from build123d import *

# Parameters (mm, degrees)
F0_W     = 50.8
F0_H     = 736.6
F1_DEPTH = 609.6
F2_W     = 685.8
F2_H     = 558.8
F3_DEPTH = 50.8
F4_W     = 25.4
F4_H     = 609.6
F5_DEPTH = 50.8


with BuildPart() as f1:
    # F0 (on Top) → F1 (new body)
    with BuildSketch(Plane.XY):
        with Locations((-589.687777, 189.852441)):
            Rectangle(F0_W, F0_H)
    extrude(amount=F1_DEPTH)

    # F2 (on face) → F3 (cut)
    with BuildSketch(Plane(origin=(-615.087777, 0, 0), x_dir=(0, -1, 0), z_dir=(-1, 0, 0))):
        with Locations((-189.852441, 304.8)):
            Rectangle(F2_W, F2_H)
    extrude(amount=-F3_DEPTH, mode=Mode.SUBTRACT)

    # F4 (on face) → F5 (cut)
    with BuildSketch(Plane(origin=(-615.087777, 0, 0), x_dir=(0, -1, 0), z_dir=(-1, 0, 0))):
        with Locations((165.747559, 304.8)):
            Rectangle(F4_W, F4_H)
    extrude(amount=-F5_DEPTH, mode=Mode.SUBTRACT)


solid = f1.part
Design review of the part built by this model. Coordinates are the model's own, in mm. A direction names the side the tool comes from. Round coordinates to 2 decimals unless told otherwise and drop trailing zeros. Order: outer loops, then holes, each group sorted by start corner. A loop starts at its lowest first (then second) coordinate and runs counter-clockwise, first axis right, second up.
1) Consider section A-A (y = 333). State the section outline as (x, z) points.
The answers:
outline: (-615.09, 0) - (-564.29, 0) - (-564.29, 25.4) - (-615.09, 25.4) - close; (-615.09, 584.2) - (-564.29, 584.2) - (-564.29, 609.6) - (-615.09, 609.6) - close
2) Consider section B-B (x = -574.5). State the section outline as (y, z) points.
The answers:
outline: (-153.05, 0) - (558.15, 0) - (558.15, 609.6) - (-153.05, 609.6) - (-153.05, 584.2) - (532.75, 584.2) - (532.75, 25.4) - (-153.05, 25.4) - close
3) Machinability: for faces 1 (the flat face through (-615.088, 543, 303)), 2 (the flat face through (-590, 532.752, 301)), which of the approach directions +Z, -Z, +X, -X, +Y, -Y give a long, thin tool a straight path to every point of the face, cutting with its end or side? Answer none if there is none.
The answers:
face 1: +Z, -Z, -X, +Y, -Y
face 2: +X, -X, -Y
4) Clearance check with a flat-ended pin moving along its axis: pin 1 Ø6 at (x, z) = (-595.5, 396) entering from -Y. State where the tip first meets the part, or that it passes through.
The answers:
pin 1: stops at y = 532.75
5) For L1, parallel to Z at x = -575.5, y = 323.5; L2, parallel to Y at x = -592.5, z = 379.5, list the stretches that pass through material, from the lowest coordinate up.
The answers:
L1: z = 0 to 25.4, 584.2 to 609.6
L2: y = 532.75 to 558.15
6) Draft analysis for pull direction Z (two halves, no side actions). For faces 3 (the flat face through (-590, 208, 609.6)), 4 (the flat face through (-590, 195, 584.2)), 5 (the flat face through (-590, 195, 25.4)), 6 (the flat face through (-590, -153.048, 13)), state which applies: released by +Z, released by -Z, zero draft, split by the parting line, or undercut.
The answers:
face 3: released by +Z
face 4: undercut
face 5: undercut
face 6: zero draft
7) Consider section C-C (z = 403.5). State the section outline as (x, y) points.
The answers:
outline: (-615.09, 532.75) - (-564.29, 532.75) - (-564.29, 558.15) - (-615.09, 558.15) - close
